from build123d import *

# Parameters (mm, degrees)
F0_R     = 1
F1_DEPTH = 5


# Not quite as in the source:
# - ends of sketch curves that miss each other by under 0.0002 mm in the source are joined


with BuildPart() as f1:
    # F0 (on Top) → F1 (new body)
    with BuildSketch(Plane.XY):
        with BuildLine():
            add(Edge.make_bspline(
                [(12.5000001863, 30.3108888098), (7.72521306, 19.685755152), (28.7444061302, 17.0137217111), (30.0000001863, -3.226e-07)],
                knots=[0, 0, 0, 0, 35, 35, 35, 35], degree=3))
            ThreePointArc((12.5000001863, 30.3108888098), (-0.3108891325, 17.5), (-5, 0))
            add(Edge.make_bspline(
                [(-5, 0), (1.8142421031, -9.4476537779), (14.6378874779, 7.4194846675), (30.0000001863, -3.226e-07)],
                knots=[0, 0, 0, 0, 35, 35, 35, 35], degree=3))
        make_face()
        Circle(F0_R, mode=Mode.SUBTRACT)
        with BuildLine():
            ThreePointArc((3.1497091277, 4.3973755592), (1.867996364, 3.7997030808), (1.2703238856, 5.0814158445))
            ThreePointArc((1.2703238856, 5.0814158445), (2.5786627167, 9.9642028495), (3.0192378757, 15.0000000022))
            ThreePointArc((3.0192378757, 15.0000000022), (4.019237875, 16.0000000029), (5.0192378757, 15.0000000036))
            ThreePointArc((5.0192378757, 15.0000000036), (4.548278223, 9.6169064956), (3.1497091277, 4.3973755592))
        make_face(mode=Mode.SUBTRACT)
    extrude(amount=F1_DEPTH)


solid = f1.part
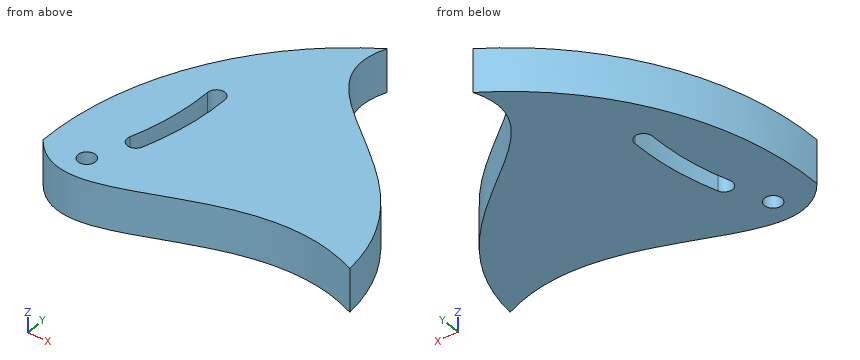
Geometry check sheet. Reference: the model listing, model coordinates, mm. Round coordinates to 2 decimals unless told otherwise and drop trailing zeros.
Item 1: Gauge pin test, flat ends, axial feed: pin 1 (1 mm diameter, centred on x = 24.5, z = 2.5, fed in from +Y); pin 2 (3 mm diameter, centred on y = 19.5, z = 1, fed in from -X); pin 3 (1 mm diameter, centred on x = 8, z = 2.5, fed in from +Y). Record the tip position at first contact, or that the pin passes through.
Item 2: Cross-section at A-A on z = 1.1. Count the separate pieces of the cut face and the enclosed holes in it, then the cut area to 3 significant figures.
Item 3: Thickness scan on line 1 (Y direction, x = 0, z = 1.65); line 2 (Y direction, x = -2, z = 3.65); line 3 (X direction, y = 17, z = 0.5). Record the ranges inside material, lowest first.
Answer sheet:
1. pin 1: stops at y = 12.89
1. pin 2: stops at x = -0.02
1. pin 3: stops at y = 27.62
2. separate pieces: 1
2. enclosed holes: 2
2. area: 614 mm2
3. line 1: y = -2.94 to -1, 1 to 18.03
3. line 2: y = -2.48 to 14.18
3. line 3: x = -0.59 to 19.63
